from build123d import *

# Parameters (mm, degrees)
F0_W      = 85
F0_H      = 85
F0_R      = 2
F3_DEPTH  = 18.5
F4_DEPTH  = 14
F5_R      = 5
F6_R      = 3
F7_R      = 1
F8_R      = 3.1
F9_DEPTH  = 3.1
F10_R     = 3.1
F11_DEPTH = 3.1
F12_R     = 3.1
F13_DEPTH = 3.1
F14_R     = 3.1
F15_DEPTH = 3.1
F16_DEPTH = 1
F17_ANGLE = 180


# Not quite as in the source:
# - a feature names something its author has since deleted; it is built from what else it names


with BuildPart() as f3:
    # F0 (on Top) → F3 (new body)
    with BuildSketch(Plane.XY):
        Rectangle(F0_W, F0_H)
        with BuildLine():
            ThreePointArc((-33, 12), (-32.1213203436, 14.1213203436), (-30, 15))
            Line((-30, 15), (30, 15))
            ThreePointArc((30, 15), (32.1213203436, 14.1213203436), (33, 12))
            Line((33, 12), (33, -30))
            ThreePointArc((33, -30), (32.1213203436, -32.1213203436), (30, -33))
            Line((30, -33), (-30, -33))
            ThreePointArc((-30, -33), (-32.1213203436, -32.1213203436), (-33, -30))
            Line((-33, -30), (-33, 12))
        make_face(mode=Mode.SUBTRACT)
        with BuildLine():
            ThreePointArc((-33, 30), (-32.1213203436, 32.1213203436), (-30, 33))
            Line((-30, 33), (30, 33))
            ThreePointArc((30, 33), (32.1213203436, 32.1213203436), (33, 30))
            Line((33, 30), (33, 24))
            ThreePointArc((33, 24), (32.1213203436, 21.8786796564), (30, 21))
            Line((30, 21), (-30, 21))
            ThreePointArc((-30, 21), (-32.1213203436, 21.8786796564), (-33, 24))
            Line((-33, 24), (-33, 30))
        make_face(mode=Mode.SUBTRACT)
        with Locations((0, 37.75)):
            Circle(F0_R, mode=Mode.SUBTRACT)
        with BuildLine():
            Line((30, 15), (-30, 15))
            ThreePointArc((-30, 15), (-32.1213203436, 14.1213203436), (-33, 12))
            Line((-33, 12), (-33, -30))
            ThreePointArc((-33, -30), (-32.1213203436, -32.1213203436), (-30, -33))
            Line((-30, -33), (30, -33))
            ThreePointArc((30, -33), (32.1213203436, -32.1213203436), (33, -30))
            Line((33, -30), (33, 12))
            ThreePointArc((33, 12), (32.1213203436, 14.1213203436), (30, 15))
        make_face()
        with BuildLine():
            Line((30, 33), (-30, 33))
            ThreePointArc((-30, 33), (-32.1213203436, 32.1213203436), (-33, 30))
            Line((-33, 30), (-33, 24))
            ThreePointArc((-33, 24), (-32.1213203436, 21.8786796564), (-30, 21))
            Line((-30, 21), (30, 21))
            ThreePointArc((30, 21), (32.1213203436, 21.8786796564), (33, 24))
            Line((33, 24), (33, 30))
            ThreePointArc((33, 30), (32.1213203436, 32.1213203436), (30, 33))
        make_face()
        with Locations((0, 37.75)):
            Circle(F0_R)
    extrude(amount=F3_DEPTH)

    # F0 (on Top) → F4 (cut)
    with BuildSketch(Plane.XY):
        with BuildLine():
            Line((30, 33), (-30, 33))
            ThreePointArc((-30, 33), (-32.1213203436, 32.1213203436), (-33, 30))
            Line((-33, 30), (-33, 24))
            ThreePointArc((-33, 24), (-32.1213203436, 21.8786796564), (-30, 21))
            Line((-30, 21), (30, 21))
            ThreePointArc((30, 21), (32.1213203436, 21.8786796564), (33, 24))
            Line((33, 24), (33, 30))
            ThreePointArc((33, 30), (32.1213203436, 32.1213203436), (30, 33))
        make_face()
        with BuildLine():
            Line((30, 15), (-30, 15))
            ThreePointArc((-30, 15), (-32.1213203436, 14.1213203436), (-33, 12))
            Line((-33, 12), (-33, -30))
            ThreePointArc((-33, -30), (-32.1213203436, -32.1213203436), (-30, -33))
            Line((-30, -33), (30, -33))
            ThreePointArc((30, -33), (32.1213203436, -32.1213203436), (33, -30))
            Line((33, -30), (33, 12))
            ThreePointArc((33, 12), (32.1213203436, 14.1213203436), (30, 15))
        make_face()
    extrude(amount=F4_DEPTH, mode=Mode.SUBTRACT)

    # F5
    f5_edges = [f3.edges().sort_by_distance(p)[0] for p in [
        (0, 42.5, 18.5),
        (-42.5, 0, 18.5),
        (0, -42.5, 18.5),
        (42.5, 0, 18.5),
        (42.5, 42.5, 9.25),
        (-42.5, 42.5, 9.25),
        (-42.5, -42.5, 9.25),
        (42.5, -42.5, 9.25),
    ]]
    fillet(f5_edges, radius=F5_R)

    # F6
    f6_edges = [f3.edges().sort_by_distance(p)[0] for p in [
        (0, 33, 14),
        (-32.12132, 32.12132, 14),
        (-33, 27, 14),
        (-32.12132, 21.87868, 14),
        (0, 21, 14),
        (32.12132, 21.87868, 14),
        (33, 27, 14),
        (32.12132, 32.12132, 14),
        (0, 15, 14),
        (-32.12132, 14.12132, 14),
        (-33, -9, 14),
        (-32.12132, -32.12132, 14),
        (0, -33, 14),
        (32.12132, -32.12132, 14),
        (33, -9, 14),
        (32.12132, 14.12132, 14),
    ]]
    fillet(f6_edges, radius=F6_R)

    # F7
    f7_edges = [f3.edges().sort_by_distance(p)[0] for p in [
        (0, 42.5, 0),
        (41.035534, 41.035534, 0),
        (-41.035534, 41.035534, 0),
        (42.5, 0, 0),
        (-42.5, 0, 0),
        (41.035534, -41.035534, 0),
        (-41.035534, -41.035534, 0),
        (0, -42.5, 0),
        (0, 15, 0),
        (-32.12132, 14.12132, 0),
        (-33, -9, 0),
        (-32.12132, -32.12132, 0),
        (0, -33, 0),
        (32.12132, -32.12132, 0),
        (33, -9, 0),
        (32.12132, 14.12132, 0),
        (0, 33, 0),
        (-32.12132, 32.12132, 0),
        (-33, 27, 0),
        (-32.12132, 21.87868, 0),
        (0, 21, 0),
        (32.12132, 21.87868, 0),
        (33, 27, 0),
        (32.12132, 32.12132, 0),
    ]]
    fillet(f7_edges, radius=F7_R)

    # F8 (on face) → F9 (cut)
    with BuildSketch(Plane.XZ.offset(42.5)):
        with Locations((0, 7)):
            Circle(F8_R)
    extrude(amount=-F9_DEPTH, mode=Mode.SUBTRACT)

    # F10 (on face) → F11 (cut)
    with BuildSketch(Plane(origin=(0, 42.5, 0), x_dir=(-1, 0, 0), z_dir=(0, 1, 0))):
        with Locations((0, 7)):
            Circle(F10_R)
    extrude(amount=-F11_DEPTH, mode=Mode.SUBTRACT)

    # F12 (on face) → F13 (cut)
    with BuildSketch(Plane(origin=(-42.5, 0, 0), x_dir=(0, -1, 0), z_dir=(-1, 0, 0))):
        with Locations((0, 7)):
            Circle(F12_R)
    extrude(amount=-F13_DEPTH, mode=Mode.SUBTRACT)

    # F14 (on face) → F15 (cut)
    with BuildSketch(Plane.YZ.offset(42.5)):
        with Locations((0, 7)):
            Circle(F14_R)
    extrude(amount=-F15_DEPTH, mode=Mode.SUBTRACT)

    # F0 (on Top) → F16 (cut)
    with BuildSketch(Plane.XY):
        with Locations((0, 37.75)):
            Circle(F0_R)
    extrude(amount=F16_DEPTH, mode=Mode.SUBTRACT)


with BuildPart() as f3_1:
    # F17: moved
    add(f3.part.rotate(Axis((0, 0, 0), (0, 1, 0)), F17_ANGLE))


solid = f3_1.part
Geometry: final body of the model. Coordinates: model frame, mm. A direction names the side the tool comes from. Give positions to 0.01 mm unless a question says otherwise; leave off trailing zeros. Write each loop counter-clockwise with the first axis right and the second up, starting at its lowest first coordinate (ties: lowest second). Pieces come first, ordered by that corner, then holes. Notation, with made-up numbers: (86.5, 65) -> (117.5, 65) arc R10 cw to (117.5, 71) -> close; hole circle Ø8 at (29.5, -25.75). An arc over 180 degrees is marked (long way). Answer in a Markdown table with one row per item.
(1) Section query D-D on z = -7. State how many separate pieces and enclosed holes the cut face has, then the cut area to 3 significant figures.
Answers below:
| item | result |
|---|---|
| separate pieces | 1 |
| enclosed holes | 2 |
| area | 3,180 mm^2 |
(2) Ray query, line 1 along Y through (x, z) = (-10.5, -8.75); line 2 along X through (y, z) = (7.5, -10); line 3 along Y through (x, z) = (-32, -9.5). Return the intervals inside material, ascending. Write a range as [from, to].
Answers below:
| item | result |
|---|---|
| line 1 | [-42.5, -33], [15, 21], [33, 42.5] |
| line 2 | [-42.5, -33], [33, 42.5] |
| line 3 | [-42.5, -32.24], [14.24, 21.76], [32.24, 42.5] |
(3) Pin query (flat end, axial travel): pin 1 (3.5 mm diameter, centred on x = 0, y = 37.75, fed in from +Z); pin 2 (4 mm diameter, centred on x = 8.5, y = 3, fed in from +Z); pin 3 (12 mm diameter, centred on x = -19, y = 9.5, fed in from +Z). Return the tip coordinate at first contact, or that it passes through.
Answers below:
| item | result |
|---|---|
| pin 1 | z = -1 |
| pin 2 | z = -14 |
| pin 3 | z = -0.13 |
(4) Set-up query: faces 4 (the flat face through (1, 42.5, -11)), 5 (the cylindrical face through (-40.972, 2.957, -7.931)), 6 (the flat face through (-33, 27, -6)). Return all of +Z, -Z, +X, -X, +Y, -Y with unobstructed straight access to the full face (end or side cutting, diameter ignored); none if empty.
Answers below:
| item | result |
|---|---|
| face 4 | +Z, -Z, +X, -X, +Y |
| face 5 | -X |
| face 6 | +Z |
(5) Section query B-B on y = 11. Return loops of the section in (x, z), then the cut area to 3 significant figures.
Answers below:
| item | result |
|---|---|
| outline | (-42.5, -13.5) arc R5 ccw to (-37.5, -18.5) -> (37.5, -18.5) arc R5 ccw to (42.5, -13.5) -> (42.5, -1) arc R1 ccw to (41.5, 0) -> (34, 0) arc R1 ccw to (33, -1) -> (33, -11) arc R3 cw to (30, -14) -> (-30, -14) arc R3 cw to (-33, -11) -> (-33, -1) arc R1 ccw to (-34, 0) -> (-41.5, 0) arc R1 ccw to (-42.5, -1) -> close |
| area | 641 mm^2 |
(6) Section query A-A on x = -15.5. Return loops of the section in (y, z).
Answers below:
| item | result |
|---|---|
| outline | (-42.5, -13.5) arc R5 ccw to (-37.5, -18.5) -> (37.5, -18.5) arc R5 ccw to (42.5, -13.5) -> (42.5, -1) arc R1 ccw to (41.5, 0) -> (34, 0) arc R1 ccw to (33, -1) -> (33, -11) arc R3 cw to (30, -14) -> (24, -14) arc R3 cw to (21, -11) -> (21, -1) arc R1 ccw to (20, 0) -> (16, 0) arc R1 ccw to (15, -1) -> (15, -11) arc R3 cw to (12, -14) -> (-30, -14) arc R3 cw to (-33, -11) -> (-33, -1) arc R1 ccw to (-34, 0) -> (-41.5, 0) arc R1 ccw to (-42.5, -1) -> close |
(7) Section query C-C on z = -15.5. Return loops of the section in (x, y), then the cut area to 3 significant figures.
Answers below:
| item | result |
|---|---|
| outline | (-42.08, -37.5) arc R4.58 ccw to (-37.5, -42.08) -> (37.5, -42.08) arc R4.58 ccw to (42.08, -37.5) -> (42.08, 37.5) arc R4.58 ccw to (37.5, 42.08) -> (-37.5, 42.08) arc R4.58 ccw to (-42.08, 37.5) -> close |
| area | 7,070 mm^2 |
(8) Draft query along Y for faces 1 (the cylindrical face through (-41, 0.52, -17.07)), 2 (the flat face through (0, 39.4, -7)), 3 (the flat face through (33, 27, -6)). Return one class per face: +Y half, -Y half, draft (parallel to the pull), parting line (faces both ways), or undercut.
Answers below:
| item | result |
|---|---|
| face 1 | draft |
| face 2 | +Y half |
| face 3 | undercut |
